The listing builds one solid part. Answer for the finished solid, in the listing's coordinates (mm). A direction names the side the tool comes from. Round coordinates to 2 decimals unless told otherwise and drop trailing zeros. Order: outer loops, then holes, each group sorted by start corner. A loop starts at its lowest first (then second) coordinate and runs counter-clockwise, first axis right, second up. Notation, with made-up numbers: M 0.25,51.25 L 19.25,51.25 A13 cw 19.25,61.25 Z; hole C -4.5,1.25 d10. An arc over 180 degrees is marked long. Put each result on its own line as item: value. Start each with the question number.
1. Which of the six approach directions +Z, -Z, +X, -X, +Y, -Y give full straight-line access (tool end or side, diameter ignored) to faces 5 (the face through (5.4, 5.5, 0)), 6 (the face through (5.42, -4.46, -3.22)), 7 (the face through (5.4, -0.9, 2.86))?
2. The part is cut by section A-A (y = 0). Give the vertices of the cut face in (x, z).
3. Each of these flat-tipped pins is pushed along its axis until it touches: pin 1 Ø1 at (x, y) = (3, 3) entering from +Z; pin 2 Ø6 at (x, y) = (4.5, 2) entering from +Z; pin 3 Ø5 at (y, z) = (2, 0) entering from +X; pin 4 Ø8 at (x, y) = (11, -5) entering from -Z. Where does it stop, or does it pass through?
4. Consider line 1 (X direction, y = -7, z = -2.75); line 2 (Y direction, x = 4, z = 0); line 3 (Y direction, x = 4, z = -5.75). Determine where each line is inside the solid, lowest interval first.
5. The mould has two halves that part along X. Classify faces 1 (the face through (5.423, -4.438, 3.247)), 2 (the face through (5.42, -0.56, 5.47)), 3 (the face through (-2, 0, 4)), 4 (the face through (-1.01, 8.923, -1.172)): +X half, -X half, draft (parallel to the pull), parting line (faces both ways), or undercut.
from build123d import *

# Parameters (mm, degrees)
CHAMFER_1_SIZE           = 1
SKETCH_4_W               = 2
SKETCH_4_H               = 1.440270842
CUT_EXTRUDE_1_DEPTH      = 23.179036994
CUT_EXTRUDE_2_REACH      = 24.179
PATTERN_CIRCULAR_3_COUNT = 15
SKETCH_7_R               = 3
CUT_EXTRUDE_3_DEPTH      = 23.173117564
EXTRUDE_START            = 2
SKETCH_9_R               = 9
SKETCH_9_R_2             = 3
EXTRUDE_1_DEPTH          = 2
SKETCH_10_R              = 9
SKETCH_10_R_2            = 3
EXTRUDE_2_DEPTH          = 2
CHAMFER_2_SIZE           = 0.3


with BuildPart() as part:
    # 草图1 → 旋转1 (revolve)
    with BuildSketch(Plane.XY, mode=Mode.PRIVATE) as revolve_1_sk:
        Polygon((0, 1.3558), (0, 6.779), (11, 6.779), (11, 2.7116), (20, 2.7116), (20, 1.3558), align=None)
    revolve(revolve_1_sk.sketch.rotate(Axis((0, 0, 0), (1, 0, 0)), 90), axis=Axis((0, 0, 0), (1, 0, 0)))

    # 倒角1
    chamfer_1_edges = [part.edges().sort_by_distance(p)[0] for p in [
        (20, 0, -1.3558),
        (0, 0, -1.3558),
    ]]
    chamfer(chamfer_1_edges, length=CHAMFER_1_SIZE)

    # 草图4 → 切除-拉伸1 (cut, through all)
    with BuildSketch(Plane.ZY):
        with Locations((0, 1.635664579)):
            Rectangle(SKETCH_4_W, SKETCH_4_H)
    extrude(amount=-CUT_EXTRUDE_1_DEPTH, mode=Mode.SUBTRACT)

    # 草图6 → 切除-拉伸2 (cut, up to next)
    with BuildSketch(Plane(origin=(0, 0, 0), x_dir=(0, 0, -1), z_dir=(1, 0, 0)), mode=Mode.PRIVATE) as cut_extrude_2_sk1:
        with BuildLine():
            Line((0.921029279, 6.443168288), (0.903216998, 6.298098898))
            ThreePointArc((0.903216998, 6.298098898), (0, 5.499), (-0.903216998, 6.298098898))
            Line((-0.903216998, 6.298098898), (-0.921029279, 6.443168288))
            ThreePointArc((-0.921029279, 6.443168288), (-1.025205225, 6.62105106), (-1.226117469, 6.667194084))
            ThreePointArc((-1.226117469, 6.667194084), (-1.353747907, 6.642454938), (-1.480880455, 6.615272789))
            Line((-1.480880455, 6.615272789), (-1.677528444, 8.216842132))
            ThreePointArc((-1.677528444, 8.216842132), (0, 8.386333901), (1.677528444, 8.216842132))
            Line((1.677528444, 8.216842132), (1.480880455, 6.615272789))
            ThreePointArc((1.480880455, 6.615272789), (1.353747907, 6.642454938), (1.226117469, 6.667194084))
            ThreePointArc((1.226117469, 6.667194084), (1.025205225, 6.62105106), (0.921029279, 6.443168288))
        make_face()
    cut_extrude_2_tool1 = extrude(cut_extrude_2_sk1.sketch, amount=CUT_EXTRUDE_2_REACH, mode=Mode.PRIVATE) & part.part
    cut_extrude_2 = cut_extrude_2_tool1.solids().sort_by_distance((0, 7.172733, 0))[0]
    add(cut_extrude_2, mode=Mode.SUBTRACT)

    # 阵列(圆周)3: 切除-拉伸2 ×15 about axis
    pattern_circular_3_axis = Axis((0, 0, 0), (1, 0, 0))
    for i in range(1, PATTERN_CIRCULAR_3_COUNT):
        add(cut_extrude_2.rotate(pattern_circular_3_axis, i * 360 / PATTERN_CIRCULAR_3_COUNT), mode=Mode.SUBTRACT)

    # 草图7 → 切除-拉伸3 (cut, through all)
    with BuildSketch(Plane.ZY):
        Circle(SKETCH_7_R)
    extrude(amount=-CUT_EXTRUDE_3_DEPTH, mode=Mode.SUBTRACT)

    # 草图9 → 凸台-拉伸1 (add)
    with BuildSketch(Plane.ZY.offset(EXTRUDE_START)):
        Circle(SKETCH_9_R)
        Circle(SKETCH_9_R_2, mode=Mode.SUBTRACT)
    extrude(amount=-EXTRUDE_1_DEPTH)

    # 草图10 → 凸台-拉伸2 (add)
    with BuildSketch(Plane(origin=(11, 0, 0), x_dir=(0, 0, -1), z_dir=(1, 0, 0))):
        with Locations(Location((0, 0, 0), (0, 0, 180))):
            Circle(SKETCH_10_R)
        with Locations(Location((0, 0, 0), (0, 0, 180))):
            Circle(SKETCH_10_R_2, mode=Mode.SUBTRACT)
    extrude(amount=EXTRUDE_2_DEPTH)

    # 倒角2
    chamfer_2_edges = [part.edges().sort_by_distance(p)[0] for p in [
        (-2, 0, -9),
        (0, 0, -9),
        (13, 0, -9),
        (11, 0, -9),
    ]]
    chamfer(chamfer_2_edges, length=CHAMFER_2_SIZE)


solid = part.part
Resolved:
1. face 5: +Y
1. face 6: none
1. face 7: +X, -X
2. outline: M -2,-8.7 L -1.7,-9 L -0.3,-9 L 0,-8.7 L 0,-5.76 L 11,-5.76 L 11,-8.7 L 11.3,-9 L 12.7,-9 L 13,-8.7 L 13,-3 L -2,-3 Z; M -2,3 L 13,3 L 13,8.7 L 12.7,9 L 11.3,9 L 11,8.7 L 11,5.76 L 0,5.76 L 0,8.7 L -0.3,9 L -1.7,9 L -2,8.7 Z
3. pin 1: z = 5.99
3. pin 2: z = 6.76
3. pin 3: x = 13
3. pin 4: z = -8.94
4. line 1: -2 to 0, 11 to 13
4. line 2: -6.78 to -3, 3 to 5.5
4. line 3: -2.32 to -1.33, -0.01 to 1.14, 2.82 to 3.58
5. face 1: undercut
5. face 2: undercut
5. face 3: -X half
5. face 4: draft
